```python
from build123d import *

# Parameters (mm, degrees)
F0_W     = 31.4
F0_H     = 7.4
F0_R     = 3
F1_DEPTH = 3.95
F0_R_2   = 2.499
F2_DEPTH = 3.45
F3_R     = 3.69999


# Not quite as in the source:
# - a fillet or chamfer is up to 0.001 mm smaller than in the source, because OpenCascade refuses the exact size


with BuildPart() as f1:
    # F0 (on Front) → F1 (new body, symmetric)
    with BuildSketch(Plane.XZ):
        Rectangle(F0_W, F0_H)
        with BuildLine():
            ThreePointArc((-12.9, 2.8618176043), (-12, 3), (-11.1, 2.8618176043))
            Line((-11.1, 2.8618176043), (-11.1, 0.9))
            Line((-11.1, 0.9), (-9.1381823957, 0.9))
            ThreePointArc((-9.1381823957, 0.9), (-9, 0), (-9.1381823957, -0.9))
            Line((-9.1381823957, -0.9), (-11.1, -0.9))
            Line((-11.1, -0.9), (-11.1, -2.8618176043))
            ThreePointArc((-11.1, -2.8618176043), (-12, -3), (-12.9, -2.8618176043))
            Line((-12.9, -2.8618176043), (-12.9, -0.9))
            Line((-12.9, -0.9), (-14.8618176043, -0.9))
            ThreePointArc((-14.8618176043, -0.9), (-15, 0), (-14.8618176043, 0.9))
            Line((-14.8618176043, 0.9), (-12.9, 0.9))
            Line((-12.9, 0.9), (-12.9, 2.8618176043))
        make_face(mode=Mode.SUBTRACT)
        with Locations((-4, 0)):
            Circle(F0_R, mode=Mode.SUBTRACT)
        with Locations((4, 0)):
            Circle(F0_R, mode=Mode.SUBTRACT)
        with Locations((12, 0)):
            Circle(F0_R, mode=Mode.SUBTRACT)
    extrude(amount=F1_DEPTH, both=True)

    # F0 (on Front) → F2 (join, symmetric)
    with BuildSketch(Plane.XZ):
        with Locations((-4, 0)):
            Circle(F0_R)
        with Locations((-4, 0)):
            Circle(F0_R_2, mode=Mode.SUBTRACT)
        with Locations((4, 0)):
            Circle(F0_R)
        with Locations((4, 0)):
            Circle(F0_R_2, mode=Mode.SUBTRACT)
        with Locations((12, 0)):
            Circle(F0_R)
        with Locations((12, 0)):
            Circle(F0_R_2, mode=Mode.SUBTRACT)
    extrude(amount=F2_DEPTH, both=True)

    # F3 (radius 3.7 in the source; OpenCascade refuses exactly that, so slightly less here)
    f3_edges = [f1.edges().sort_by_distance(p)[0] for p in [
        (-15.7, 0, 3.7),
        (-15.7, 0, -3.7),
        (15.7, 0, 3.7),
        (15.7, 0, -3.7),
    ]]
    fillet(f3_edges, radius=F3_R)


solid = f1.part
```
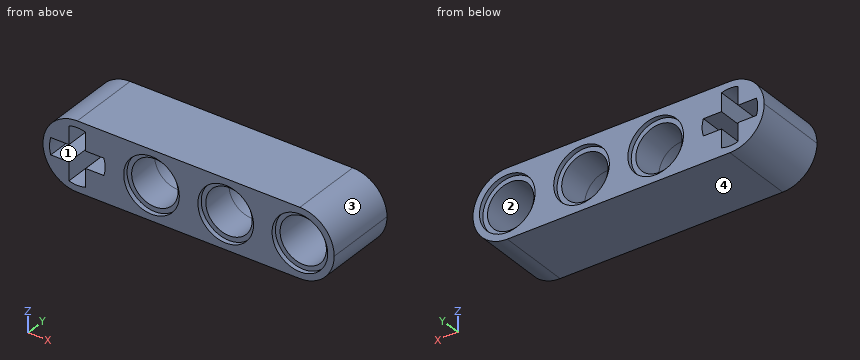
Read the model definition and answer for the solid it produces. Units are mm, in the model's axes. Face numbers are marked on the shaded views. Give positions to 0.01 mm unless a question says otherwise; leave off trailing zeros. Loops run counter-clockwise (first coordinate to the right, second up) from the corner with the lowest first, then second, coordinate; pieces in that order, holes last.
Item 1: Each of these flat-tipped pins is pushed along its axis until it touches: pin 1 Ø1.5 at (x, z) = (11.5, 0) entering from -Y; pin 2 Ø0.6 at (y, z) = (0.5, -2) entering from -X; pin 3 Ø3 at (x, z) = (-3, 0.5) entering from +Y; pin 4 Ø1 at (y, z) = (-0.5, 2) entering from +X. Where does it stop, or does it pass through?
Item 2: Find the intervals of material crossed by line 1 along X through (y, z) = (-3.25, -0.75); line 2 along Z through (x, y) = (4, -1.55); line 3 along X through (y, z) = (-2.25, -1), in increasing order.
Item 3: The mould has two halves that part along Z. Classify the marked faces 1, 2, 3 and 4: released by +Z, released by -Z, zero draft, split by the parting line, or undercut.
Item 4: The part is cut by section C-C (x = -5). Write down the section's boundary in (y, z).
Item 5: The part is cut by section A-A (y = -1.25). Give the number of separate pieces and of enclosed holes in the cut face, and give its area (3 significant figures).
Item 6: The part is cut by section B-B (x = 3.5). Write down the section's boundary in (y, z), and give its area (3 significant figures).
Taken from the geometry:
1. pin 1: passes through
1. pin 2: stops at x = -15.29
1. pin 3: stops at y = 3.45
1. pin 4: stops at x = 15.38
2. line 1: x = -15.62 to -14.9, -9.1 to -6.38, -1.62 to 1.62, 6.38 to 9.62, 14.38 to 15.62
2. line 2: z = -3.7 to -2.5, 2.5 to 3.7
2. line 3: x = -15.56 to -12.9, -11.1 to -6.29, -1.71 to 1.71, 6.29 to 9.71, 14.29 to 15.56
3. face 1: undercut
3. face 2: undercut
3. face 3: released by +Z
3. face 4: released by -Z
4. outline: (-3.95, -3.7) - (3.95, -3.7) - (3.95, -2.83) - (3.45, -2.83) - (3.45, -2.29) - (-3.45, -2.29) - (-3.45, -2.83) - (-3.95, -2.83) - close; (-3.95, 2.83) - (-3.45, 2.83) - (-3.45, 2.29) - (3.45, 2.29) - (3.45, 2.83) - (3.95, 2.83) - (3.95, 3.7) - (-3.95, 3.7) - close
5. separate pieces: 1
5. enclosed holes: 4
5. area: 144 mm2
6. outline: (-3.95, -3.7) - (3.95, -3.7) - (3.95, -2.96) - (3.45, -2.96) - (3.45, -2.45) - (-3.45, -2.45) - (-3.45, -2.96) - (-3.95, -2.96) - close; (-3.95, 2.96) - (-3.45, 2.96) - (-3.45, 2.45) - (3.45, 2.45) - (3.45, 2.96) - (3.95, 2.96) - (3.95, 3.7) - (-3.95, 3.7) - close
6. area: 18.8 mm2
